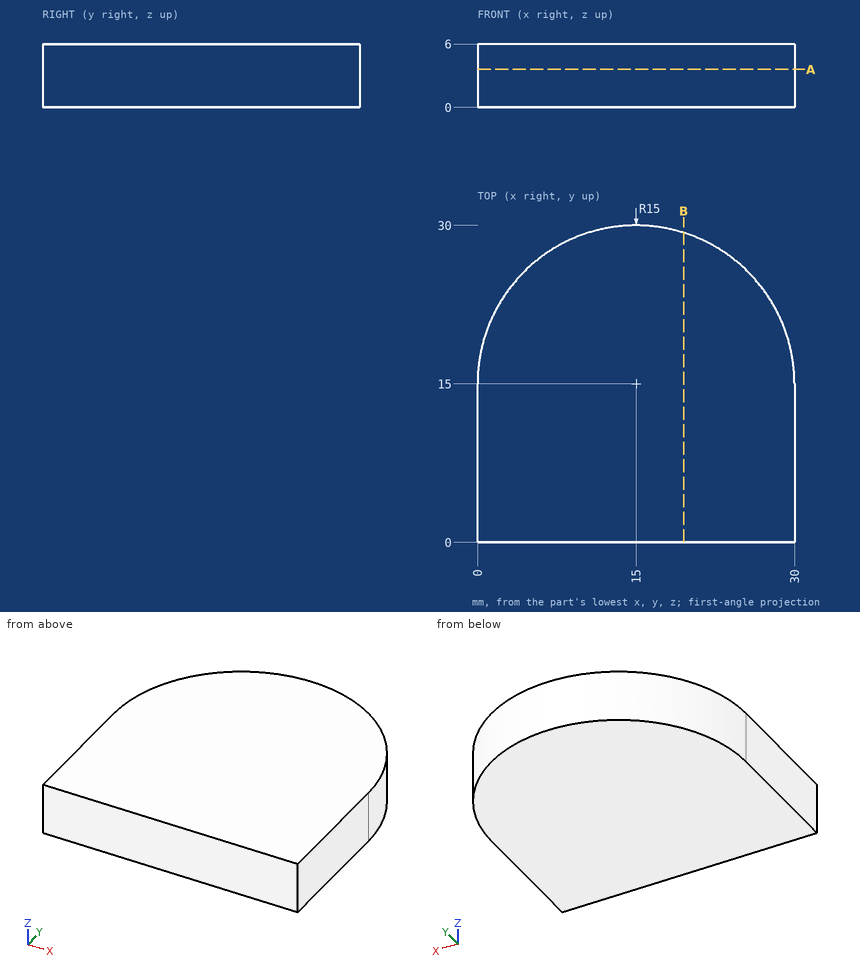
Geometry check sheet. Reference: drawing and pictorial views, mm from the part's lowest x, y, z. Coordinates: 2 decimals unless noted, no trailing zeros. Order: outer loops, then holes, each group sorted by start corner. A loop starts at its lowest first (then second) coordinate and runs counter-clockwise, first axis right, second up. Notation, with made-up numbers: (-6, 84) -> (53, 84) arc R23 ccw to (53, 106) -> close; hole circle Ø8 at (-17, 72.25). An arc over 180 degrees is marked (long way). Write item = value, one per line. Start each with the question number.
1) Cross-section at A-A (z = 3.6). Enter the section's corners in (x, y), then the cut area to 3 significant figures.
2) Material ranges on L1, parallel to Y at x = 15.25, z = 3.4; L2, parallel to Y at x = 5.75, z = 3.3; L3, parallel to X at y = 18.75, z = 5.35, recorded low to high.
3) Cross-section at B-B (x = 19.5). Enter the section's corners in (y, z).
Ans:
q1.outline = (0, 0) -> (30, 0) -> (30, 15) arc R15 ccw to (0, 15) -> close
q1.area = 803 mm²
q2.L1 = 0 to 30
q2.L2 = 0 to 26.81
q2.L3 = 0.48 to 29.52
q3.outline = (0, 0) -> (29.31, 0) -> (29.31, 6) -> (0, 6) -> close
